Part print with two shaded views. Sizes in mm from the minimum x, y, z corner. Round coordinates to 2 decimals unless told otherwise and drop trailing zeros. Write each loop counter-clockwise with the first axis right and the second up, starting at its lowest first coordinate (ties: lowest second). Pieces come first, ordered by that corner, then holes. Notation, with made-up numbers: M 21,3.25 L 63,3.25 A14 ccw 63,10.25 Z; hole C 74.5,21 d5. An arc over 180 degrees is marked long. Use one line per item in the form item = value. Start each with the question number.
Item 1: Cut at D-D, the plane x = 2. Give the cut face in (y, z).
Item 2: Cut at C-C, the plane z = 3. Give the cut face in (x, y).
Item 3: Flat gauge pins, fed straight in: pin 1 Ø3 at (y, z) = (4.5, 22) entering from +X; pin 2 Ø1.5 at (x, y) = (5.5, 7) entering from +Z; pin 3 Ø2 at (x, z) = (29.5, 29) entering from +Y; pin 4 Ø18.5 at (x, y) = (17, 17) entering from -Z. Where does each tip first touch, or does it go through?
Item 4: Mould opens along X. For the marked faces 1, 2 and 3 say: +X half, -X half, draft (parallel to the pull), parting line (faces both ways), or undercut.
Item 5: Cut at A-A, the plane y = 17. Give the cut face in (x, z), then the cut area to 3 significant figures.
Item 6: Probe L1, parallel to Y at x = 17, z = 18; L2, parallel to Y at x = 16.5, z = 3; L3, parallel to X at y = 16, z = 28. List the from-to ranges inside material, lowest first.
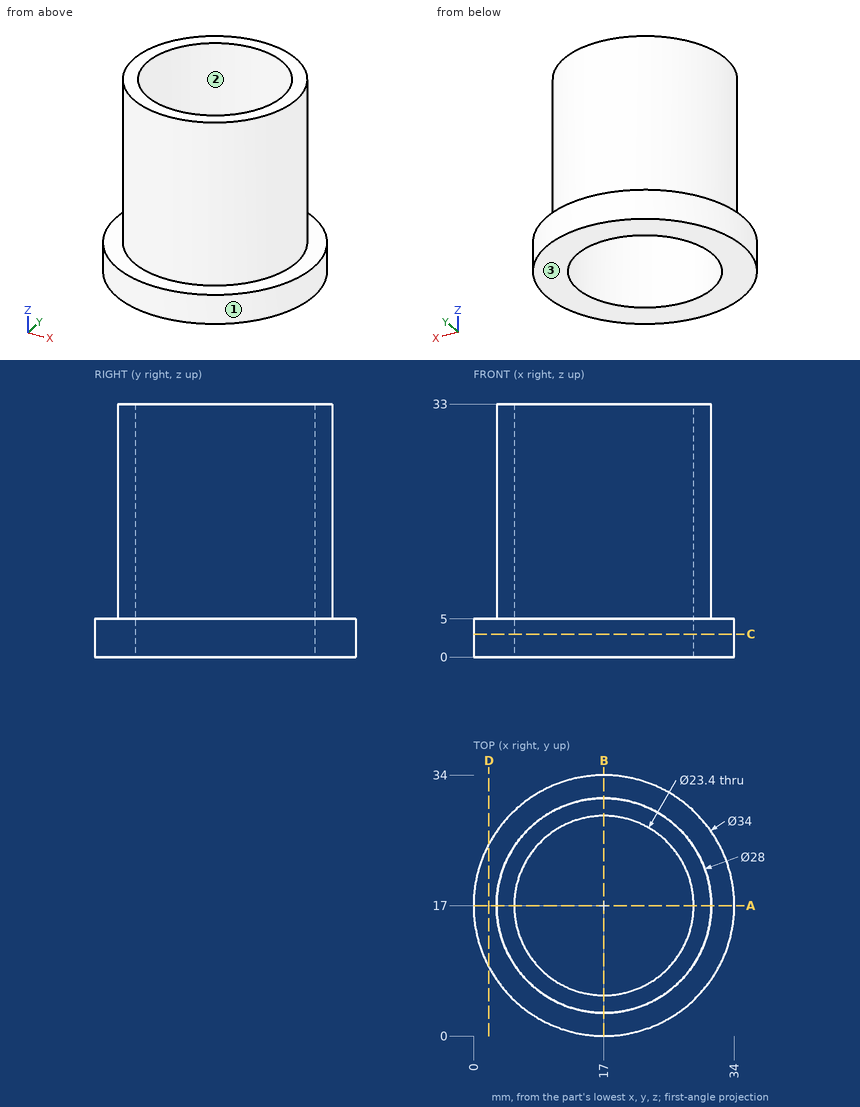
Model answer:
q1.outline = M 9,0 L 25,0 L 25,5 L 9,5 Z
q2.outline = C 17,17 d34; hole C 17,17 d23.4
q3.pin_1 = 25.66
q3.pin_2 = 5
q3.pin_3 = 24.98
q3.pin_4 = through
q4.face_1 = parting line
q4.face_2 = undercut
q4.face_3 = draft
q5.outline = M 0,0 L 5.3,0 L 5.3,33 L 3,33 L 3,5 L 0,5 Z; M 28.7,0 L 34,0 L 34,5 L 31,5 L 31,33 L 28.7,33 Z
q5.area = 182 mm²
q6.L1 = 3 to 5.3, 28.7 to 31
q6.L2 = 0.01 to 5.31, 28.69 to 33.99
q6.L3 = 3.04 to 5.34, 28.66 to 30.96
